Verification items for the finished model (mm, model axes). A direction names the side the tool comes from. Coordinates: 2 decimals unless noted, no trailing zeros. Order: outer loops, then holes, each group sorted by start corner. A loop starts at its lowest first (then second) coordinate and runs counter-clockwise, first axis right, second up. Notation, with made-up numbers: M 75.5,-20.5 L 95.5,-20.5 A16 ccw 95.5,-10.5 Z; hole C 51,-9.5 d1. An arc over 180 degrees is marked long. Return JSON: item names as keys, results as strings. Group by question number.
1. Mould release check, pull along X, two halves, no side actions. Record for faces 1 (the flat face through (63.5, 38, 1)), 2 (the flat face through (-54.133, 15.21, -25.025)), 3 (the cylindrical face through (-0.92, 60.01, 0.18)): +X half, -X half, draft (parallel to the pull), parting line (faces both ways), or undercut.
2. Section check C-C, the plane y = 15. Record the cut outline in (x, z), plus the area to 3 significant figures.
3. Set-up check for faces 4 (the flat face through (-1, 38, -12.7)), 5 (the flat face through (-44.5, 11, -22)), 6 (the flat face through (44.5, 8, 20)): record each of +Z, -Z, +X, -X, +Y, -Y from which the full face is reachable in a straight line by a thin tool's end or side.
4. Section check A-A, the plane z = -24. Record the cut outline in (x, y).
5. Section check D-D, the plane x = -52.5. Record the cut outline in (y, z), plus the area to 3 significant figures.
6. Material ranges on line 1 along X through (y, z) = (6, 16); line 2 along Z through (x, y) = (-0.5, 53.5); line 3 along X through (y, z) = (86, -6), recorded low to high.
7. Gauge pin test, flat ends, axial feed: pin 1 (1 mm diameter, centred on y = 41, z = -14.5, fed in from -X); pin 2 (12 mm diameter, centred on x = -36, y = 61, fed in from +Z). Record the tip position at first contact, or that the pin passes through.
8. Section check B-B, the plane y = 63. Record the cut outline in (x, z).
```python
from build123d import *

# Parameters (mm, degrees)
SKETCH1_W           = 127
SKETCH1_H           = 25.4
BOSS_EXTRUDE1_DEPTH = 100
SKETCH2_R           = 44.45
CUT_EXTRUDE1_DEPTH  = 30
SKETCH3_W           = 19
SKETCH3_H           = 25
BOSS_EXTRUDE2_DEPTH = 30
CUT_EXTRUDE2_DEPTH  = 140


with BuildPart() as part:
    # Sketch1 → Boss-Extrude1 (new body)
    with BuildSketch(Plane(origin=(0, 0, 0), x_dir=(1, 0, 0), z_dir=(0, 1, 0))):
        Rectangle(SKETCH1_W, SKETCH1_H)
    extrude(amount=BOSS_EXTRUDE1_DEPTH)

    # Sketch2 → Cut-Extrude1 (cut)
    with BuildSketch(Plane.XY.offset(12.7)):
        with Locations((0, 104.45)):
            Circle(SKETCH2_R)
    extrude(amount=-CUT_EXTRUDE1_DEPTH, mode=Mode.SUBTRACT)

    # Sketch3 → Boss-Extrude2 (add)
    with BuildSketch(Plane(origin=(0, 0, 0), x_dir=(1, 0, 0), z_dir=(0, 1, 0))):
        with Locations((-54, 25.2)):
            Rectangle(SKETCH3_W, SKETCH3_H)
        with Locations((54, 25.2)):
            Rectangle(SKETCH3_W, SKETCH3_H)
        with Locations((54, -25.2)):
            Rectangle(SKETCH3_W, SKETCH3_H)
        with Locations((-54, -25.2)):
            Rectangle(SKETCH3_W, SKETCH3_H)
    extrude(amount=BOSS_EXTRUDE2_DEPTH)

    # Sketch4 → Cut-Extrude2 (cut)
    with BuildSketch(Plane.ZY.offset(63.5)):
        Polygon((12.7, 30), (37.7, 0), (37.7, 30), align=None)
        Polygon((-12.7, 30), (-37.7, 0), (-37.7, 30), align=None)
    extrude(amount=-CUT_EXTRUDE2_DEPTH, mode=Mode.SUBTRACT)


solid = part.part
```
Answers follow:
{
 "1": {"face 1": "+X half", "face 2": "draft", "face 3": "undercut"},
 "2": {"outline": "M -63.5,-25.2 L -44.5,-25.2 L -44.5,-12.7 L 44.5,-12.7 L 44.5,-25.2 L 63.5,-25.2 L 63.5,25.2 L 44.5,25.2 L 44.5,12.7 L -44.5,12.7 L -44.5,25.2 L -63.5,25.2 Z", "area": "4,180 mm^2"},
 "3": {"face 4": "-Z, +Y", "face 5": "-Z, +Y, -Y", "face 6": "+Z, +Y, -Y"},
 "4": {"outline": "M -63.5,0 L -44.5,0 L -44.5,16.44 L -63.5,16.44 Z; M 44.5,0 L 63.5,0 L 63.5,16.44 L 44.5,16.44 Z"},
 "5": {"outline": "M 0,-37.7 L 30,-12.7 L 100,-12.7 L 100,12.7 L 30,12.7 L 0,37.7 Z", "area": "3,290 mm^2"},
 "6": {"line 1": "-63.5 to -44.5, 44.5 to 63.5", "line 2": "-12.7 to 12.7", "line 3": "-63.5 to -40.44, 40.44 to 63.5"},
 "7": {"pin 1": "through", "pin 2": "z = 12.7"},
 "8": {"outline": "M -63.5,-12.7 L -16.05,-12.7 L -16.05,12.7 L -63.5,12.7 Z; M 16.05,-12.7 L 63.5,-12.7 L 63.5,12.7 L 16.05,12.7 Z"}
}
